Input: dimensioned drawing with shaded views. Units: mm. Origin: part minimum x, y, z. Round coordinates to 2 decimals unless told otherwise and drop trailing zeros. Loops run counter-clockwise (first coordinate to the right, second up) from the corner with the lowest first, then second, coordinate; pieces in that order, holes last. Notation, with made-up numbers: (80, 73.5) - (119, 73.5) arc R23 cw to (119, 109.5) - close; hole circle Ø3 at (-8, -17). An arc over 180 degrees is marked (long way). One line per question, with ' | ' between items. Start each with the question number.
1. Pin query (flat end, axial travel): pin 1 (4 mm diameter, centred on x = 6.75, z = 7.55, fed in from -Y). Return the tip coordinate at first contact, or that it passes through.
2. Cut plane B-B (z = 38.05). Return loops of the section in (x, y).
3. Ray query, line 1 (Z direction, x = 6.75, y = 8); line 2 (X direction, y = 8.25, z = 38.05); line 3 (Z direction, x = 5, y = 9.75). Return the intervals inside material, ascending.
4. Cut plane A-A (x = 37.25). Return loops of the section in (y, z).
5. Mould query, pull axis Z, two halves, no side actions, for the marked faces 1, 2 and 3. Classes: pulls with the +Z half, pulls with the -Z half, needs draft (parallel to the pull), parting line crosses it, or undercut.
6. Cut plane C-C (y = 11). Return loops of the section in (x, z).
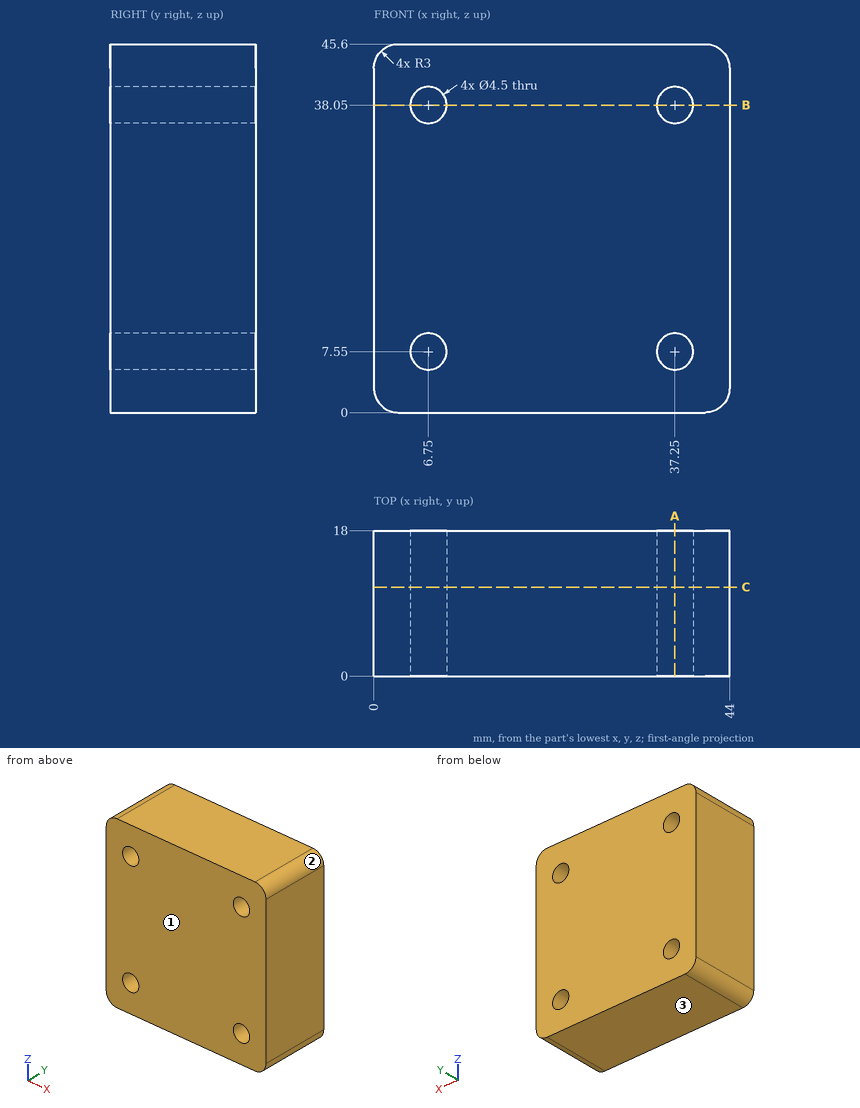
Answers follow:
1) pin 1: passes through
2) outline: (0, 0) - (4.5, 0) - (4.5, 18) - (0, 18) - close; (9, 0) - (35, 0) - (35, 18) - (9, 18) - close; (39.5, 0) - (44, 0) - (44, 18) - (39.5, 18) - close
3) line 1: z = 0 to 5.3, 9.8 to 35.8, 40.3 to 45.6 | line 2: x = 0 to 4.5, 9 to 35, 39.5 to 44 | line 3: z = 0 to 6.14, 8.96 to 36.64, 39.46 to 45.6
4) outline: (0, 0) - (18, 0) - (18, 5.3) - (0, 5.3) - close; (0, 9.8) - (18, 9.8) - (18, 35.8) - (0, 35.8) - close; (0, 40.3) - (18, 40.3) - (18, 45.6) - (0, 45.6) - close
5) face 1: needs draft | face 2: pulls with the +Z half | face 3: pulls with the -Z half
6) outline: (0, 3) arc R3 ccw to (3, 0) - (41, 0) arc R3 ccw to (44, 3) - (44, 42.6) arc R3 ccw to (41, 45.6) - (3, 45.6) arc R3 ccw to (0, 42.6) - close; hole circle Ø4.5 at (6.75, 7.55); hole circle Ø4.5 at (6.75, 38.05); hole circle Ø4.5 at (37.25, 7.55); hole circle Ø4.5 at (37.25, 38.05)
